Model file for the job. Use its own axes, mm. Face numbers are marked on the shaded views. A direction names the side the tool comes from. Coordinates: 2 decimals unless noted, no trailing zeros. Order: outer loops, then holes, each group sorted by start corner. A loop starts at its lowest first (then second) coordinate and runs counter-clockwise, first axis right, second up. Notation, with made-up numbers: (-7.75, -10.5) -> (1.25, -10.5) arc R22 cw to (1.25, 16.5) -> close; hole circle Ø7 at (29.5, 73). An arc over 180 degrees is marked (long way). Return JSON: item names as keys, results as strings. Group by question number.
1) Flat gauge pins, fed straight in: pin 1 (2 mm diameter, centred on x = -2, y = 5.5, fed in from +Z); pin 2 (1 mm diameter, centred on y = -0.5, z = 1.5, fed in from +X). Where does each tip first touch, or does it go through?
2) Cut at B-B (y = -0.5). Write the cut outline in (x, z), and give its area (3 significant figures).
3) Cut at D-D (y = 3.75). Write the cut outline in (x, z).
4) Cut at C-C (z = 0.6). Write the cut outline in (x, y), and give its area (3 significant figures).
5) Probe line 1 (Y direction, x = -0.5, z = -2.4); line 2 (Z direction, x = 0, y = 7); line 3 (X direction, y = 4.25, z = 0.15). List the from-to ranges inside material, lowest first.
6) Cut at A-A (x = 0). Write the cut outline in (y, z), and give its area (3 significant figures).
7) Which spindle directions (+Z, -Z, +X, -X, +Y, -Y) get a long thin tool onto all of the face, cutting with end or side? Do the marked faces 1 and 2. Say none if no direction does.
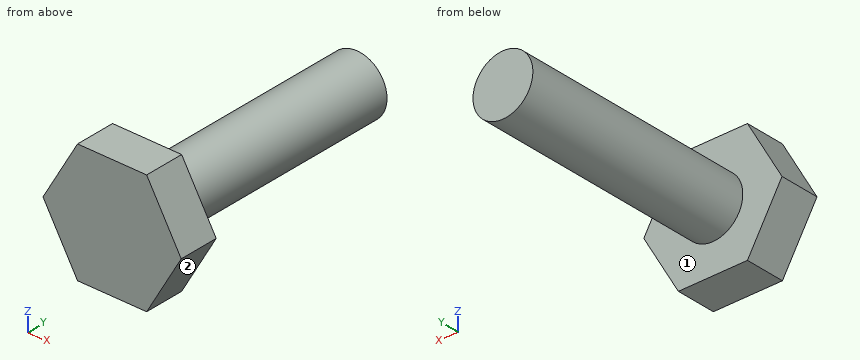
Autodesk Fusion 360 part; units mm, degrees
sketch "Sketch1" plane through (0, 0, 0) normal (0, 1, 0) x (1, 0, 0)
  circle A0 centre (0, 0) radius 1.5
  line L0 (-1.7321, 3) -> (-3.4641, 0)
  line L1 (-3.4641, 0) -> (-1.7321, -3)
  line L2 (-1.7321, -3) -> (1.7321, -3)
  line L3 (1.7321, -3) -> (3.4641, 0)
  line L4 (3.4641, 0) -> (1.7321, 3)
  line L5 (1.7321, 3) -> (-1.7321, 3)
  dimension "d1" = 3
  dimension "d2" = 6
extrude "Extrude1" add sketch "Sketch1" along normal blind 12 contours A0
extrude "Extrude2" add sketch "Sketch1" against normal blind 2 contours A0 | L0 L1 L2 L3 L4 L5
Answers below:
{
 "1": {"pin 1": "stops at z = 1.12", "pin 2": "stops at x = 2.89"},
 "2": {"outline": "(-3.46, 0) -> (-1.73, -3) -> (1.73, -3) -> (3.46, 0) -> (1.73, 3) -> (-1.73, 3) -> close", "area": "31.2 mm^2"},
 "3": {"outline": "circle Ø3 at (0, 0)"},
 "4": {"outline": "(-3.12, -2) -> (3.12, -2) -> (3.12, 0) -> (1.37, 0) -> (1.37, 12) -> (-1.37, 12) -> (-1.37, 0) -> (-3.12, 0) -> close", "area": "45.5 mm^2"},
 "5": {"line 1": "y = -2 to 0", "line 2": "z = -1.5 to 1.5", "line 3": "x = -1.49 to 1.49"},
 "6": {"outline": "(-2, -3) -> (0, -3) -> (0, -1.5) -> (12, -1.5) -> (12, 1.5) -> (0, 1.5) -> (0, 3) -> (-2, 3) -> close", "area": "48.0 mm^2"},
 "7": {"face 1": "+Y", "face 2": "-Z, +X, +Y, -Y"}
}
